Work out the finished part from the listing and answer in its coordinate system (mm). Face numbers are marked on the shaded views. Coordinates: 2 decimals unless noted, no trailing zeros. Order: outer loops, then holes, each group sorted by start corner. A loop starts at its lowest first (then second) coordinate and runs counter-clockwise, first axis right, second up. Notation, with made-up numbers: M 44,43.5 L 84,43.5 A17 cw 84,65.5 Z; hole C 67.25,-14.5 d5. An arc over 180 degrees is marked long. Use a Markdown table: item, result.
from build123d import *

# Parameters (mm, degrees)
F0_W     = 120
F0_H     = 90
F1_DEPTH = 5
F3_DEPTH = 5
F4_R     = 15
F5_DEPTH = 5
F6_R     = 3
F7_DEPTH = 5


with BuildPart() as f1:
    # F0 (on Front) → F1 (new body)
    with BuildSketch(Plane.XZ):
        Rectangle(F0_W, F0_H)
    extrude(amount=F1_DEPTH)

    # F2 (on face) → F3 (join)
    with BuildSketch(Plane.XZ.offset(5)):
        with BuildLine():
            Line((55, -18), (55, 40))
            Line((55, 40), (-45, 40))
            Line((-45, 40), (-55, 18))
            Line((-55, 18), (-55, -18))
            Line((-55, -18), (-50, -18))
            ThreePointArc((-50, -18), (-39.393398, -22.393398), (-35, -33))
            Line((-35, -33), (-35, -40))
            Line((-35, -40), (35, -40))
            Line((35, -40), (35, -33))
            ThreePointArc((35, -33), (39.393398, -22.393398), (50, -18))
            Line((50, -18), (55, -18))
        make_face()
    extrude(amount=F3_DEPTH)

    # F4 (on face) → F5 (cut)
    with BuildSketch(Plane.XZ.offset(10)):
        Circle(F4_R)
    extrude(amount=-F5_DEPTH, mode=Mode.SUBTRACT)

    # F6 (on face) → F7 (cut)
    with BuildSketch(Plane.XZ.offset(5)):
        with Locations((0, 10)):
            Circle(F6_R)
        with Locations((-6.8, 7.332121)):
            Circle(F6_R)
        with Locations((-10, 0)):
            Circle(F6_R)
        with Locations((-7.332121, -6.8)):
            Circle(F6_R)
        with Locations((0, -10)):
            Circle(F6_R)
        with Locations((6.8, -7.332121)):
            Circle(F6_R)
        with Locations((10, 0)):
            Circle(F6_R)
        with Locations((6.8, 7.332121)):
            Circle(F6_R)
    extrude(amount=-F7_DEPTH, mode=Mode.SUBTRACT)


solid = f1.part
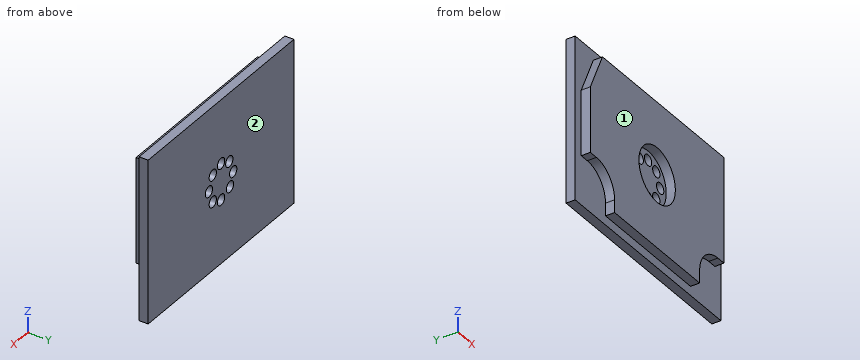
(1) A cutting plane is placed at C-C (x = -18.5). Determine the outline of the cut face in (y, z), then the cut area to 3 significant figures.
Conclusion:
| item | result |
|---|---|
| outline | M -10,-40 L -5,-40 L -5,-45 L 0,-45 L 0,45 L -5,45 L -5,40 L -10,40 Z |
| area | 850 mm2 |
(2) A cutting plane is placed at A-A (x = 0). Determine the outline of the cut face in (y, z), then the cut area to 3 significant figures.
Conclusion:
| item | result |
|---|---|
| outline | M -10,-40 L -5,-40 L -5,-45 L 0,-45 L 0,-13 L -5,-13 L -5,-15 L -10,-15 Z; M -10,15 L -5,15 L -5,13 L 0,13 L 0,45 L -5,45 L -5,40 L -10,40 Z; M -5,-7 L 0,-7 L 0,7 L -5,7 Z |
| area | 640 mm2 |
(3) Given P1, Ø5, axis at x = 6.8, z = -7.33, coming from the -Y side; P2, Ø9.5, axis at x = 0, z = -10, coming from the -Y side; P3, Ø1.5, axis at x = 51.5, y = -7, coming from the -Z side; P4, Ø5.5, axis at x = -10.5, y = -8, coming from the +Z side, each flat-ended and moving along its own axis, determine where each tip first touches the part or whether it passes through.
Conclusion:
| item | result |
|---|---|
| P1 | through |
| P2 | y = -5 |
| P3 | z = -18 |
| P4 | z = 40 |
(4) A cutting plane is placed at D-D (y = -3). Give the number of separate pieces and of enclosed holes in the cut face, then the cut area to 3 significant figures.
Conclusion:
| item | result |
|---|---|
| separate pieces | 1 |
| enclosed holes | 8 |
| area | 10,600 mm2 |
(5) A cutting plane is placed at B-B (z = 1.5). Determine the outline of the cut face in (x, y), then the cut area to 3 significant figures.
Conclusion:
| item | result |
|---|---|
| outline | M -60,-5 L -55,-5 L -55,-10 L -14.92,-10 L -14.92,-5 L -12.6,-5 L -12.6,0 L -60,0 Z; M -7.4,-5 L 7.4,-5 L 7.4,0 L -7.4,0 Z; M 12.6,-5 L 14.92,-5 L 14.92,-10 L 55,-10 L 55,-5 L 60,-5 L 60,0 L 12.6,0 Z |
| area | 949 mm2 |
(6) Determine the mould class of the marked faces 1 and 2 for opening direction Y: pulls with the +Y half, pulls with the -Y half, needs draft (parallel to the pull), parting line crosses it, or undercut.
Conclusion:
| item | result |
|---|---|
| face 1 | pulls with the -Y half |
| face 2 | pulls with the +Y half |
(7) Straight lines are drawn through the part: L1, parallel to Z at x = 0, y = -3.5; L2, parallel to Z at x = 6.8, y = -1.9; L3, parallel to Z at x = 10, y = -2.6. For each, find the intervals that lie inside material, in ascending order.
Conclusion:
| item | result |
|---|---|
| L1 | -45 to -13, -7 to 7, 13 to 45 |
| L2 | -45 to -10.33, -4.33 to 4.33, 10.33 to 45 |
| L3 | -45 to -3, 3 to 45 |
